Autodesk Inventor part; units mm, degrees
ref_plane "YZ Plane" through (0, 0, 0) normal (1, 0, 0) x (0, 1, 0)
ref_plane "XZ Plane" through (0, 0, 0) normal (0, 1, 0) x (-1, 0, 0)
ref_plane "XY Plane" through (0, 0, 0) normal (0, 0, 1) x (1, 0, 0)
sketch "Esquisse1" plane through (0, 0, 0) normal (1, 0, 0) x (0, 1, 0)
  line L0 (6.55, -1) -> (6.25, -1)
  line L1 (6.25, -1) -> (6.25, -20)
  line L2 (0, 0) -> (0, -28.3478)
  line L3 (6.55, -1) -> (9.25, -10)
  line L4 (6.55, -1) -> (6.25, 0) construction
  line L5 (9.25, -10) -> (9.25, -30)
  line L6 (6.25, -20) -> (7.25, -25)
  line L7 (7.25, -25) -> (7.25, -30)
  line L8 (7.25, -30) -> (9.25, -30)
  dimension "d0" = 12.5
  dimension "d1" = 1
  dimension "d2" = 3
  dimension "d3" = 10
  dimension "d4" = 2
  dimension "d5" = 30
  dimension "d6" = 5
  dimension "d7" = 5
  dimension "d9" = 18.5
revolve "Révolution1" add sketch "Esquisse1" angle 360 about axis through (0, 0, 0) along (0, 0, -1)
chamfer "Chanfrein1" distance 0.4 angle 45 2 edges at (0, -7.25, -30) (0, -9.25, -30)
properties part number "cardridge"
Can you work these out from the model? Positions are in its coordinate system, mm. A direction names the side the tool comes from. Coordinates: 2 decimals unless noted, no trailing zeros. Loops run counter-clockwise (first coordinate to the right, second up) from the corner with the lowest first, then second, coordinate; pieces in that order, holes last. Notation, with made-up numbers: (77.25, 41.5) -> (84.25, 41.5) arc R25 cw to (84.25, 78.5) -> close; hole circle Ø9 at (62, 69.5). An arc over 180 degrees is marked (long way). Put each result on its own line as item: value. Start each with the question number.
Q1. Thinking about a two-plate mould opening in X: for faces 1 (the face through (7, -4, -30)), 2 (the face through (-6.379, -1.417, -21.424)), 3 (the face through (-6.49, 3.38, -3.56)), which applies, pulls with the +X half, pulls with the -X half, needs draft (parallel to the pull), parting line crosses it, or undercut?
Q2. I want a section at A-A (x = 0). Write out the boundary of the cut face in (y, z), plus the area to 3 significant figures.
Q3. For faces 4 (the face through (-6.43, 3.35, -27.33)), 5 (the face through (1.88, 5.96, -10.63)), which set-ups out of +Z, -Z, +X, -X, +Y, -Y let a thin tool reach every point of the face, with its end or its side?
Q4. If I drill on line 1 (X direction, y = 0, z = -26); line 2 (X direction, y = 0, z = -11.25); line 3 (Y direction, x = -2.25, z = -4), over which ranges is the centre line in solid material (lowest first)? Write a range as [from, to].
Q5. I'm going to push flat-ended pins straight in: P1, Ø1.5, axis at x = 3, z = -13, coming from the +Y side; P2, Ø2, axis at x = -3.5, z = -24, coming from the -Y side; P3, Ø1.5, axis at x = -3.5, y = -2.5, coming from the -Z side; P4, Ø8, axis at x = 6.5, z = -26, coming from the +Y side. Where does each tip first touch, or does it pass through?
Q6. I want a section at D-D (z = -14.5). Write out the boundary of the cut face in (x, y).
Q7. I want a section at C-C (z = -28.5). Write out the boundary of the cut face in (x, y).
Taken from the geometry:
1. face 1: needs draft
1. face 2: undercut
1. face 3: parting line crosses it
2. outline: (-9.25, -29.6) -> (-8.85, -30) -> (-7.65, -30) -> (-7.25, -29.6) -> (-7.25, -25) -> (-6.25, -20) -> (-6.25, -1) -> (-6.55, -1) -> (-9.25, -10) -> close; (6.25, -20) -> (7.25, -25) -> (7.25, -29.6) -> (7.65, -30) -> (8.85, -30) -> (9.25, -29.6) -> (9.25, -10) -> (6.55, -1) -> (6.25, -1) -> close
2. area: 134 mm2
3. face 4: -Z
3. face 5: +Z, -Z
4. line 1: x = [-9.25, -7.25], [7.25, 9.25]
4. line 2: x = [-9.25, -6.25], [6.25, 9.25]
4. line 3: y = [-7.1, -5.83], [5.83, 7.1]
5. P1: stops at y = 8.97
5. P2: stops at y = -8.91
5. P3: passes through
5. P4: stops at y = 8.91
6. outline: circle Ø18.5 at (0, 0); hole circle Ø12.5 at (0, 0)
7. outline: circle Ø18.5 at (0, 0); hole circle Ø14.5 at (0, 0)
